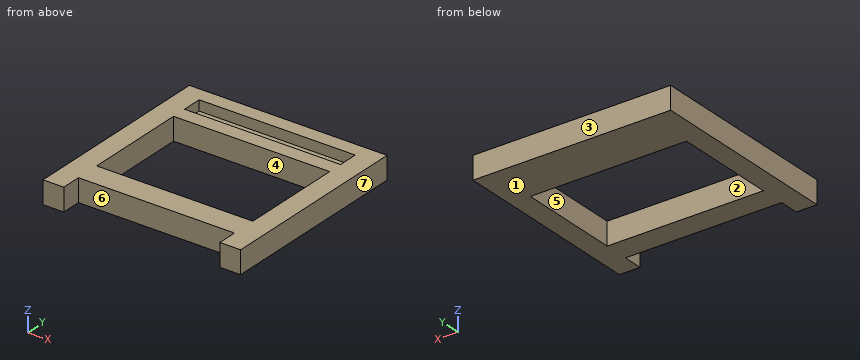
```python
from build123d import *

# Parameters (mm, degrees)
SKETCH1_W           = 15.8
SKETCH1_H           = 10.5
SKETCH1_H_2         = 2
BOSS_EXTRUDE1_DEPTH = 2.3
SKETCH1_2_W         = 15.8
SKETCH1_2_H         = 2
BOSS_EXTRUDE2_DEPTH = 1.25


with BuildPart() as part:
    # Sketch1 → Boss-Extrude1 (new body)
    with BuildSketch(Plane.XY):
        Polygon((0, 0), (0, -2), (2.1, -2), (2.1, 0), (17.9, 0), (17.9, -2), (20, -2), (20, 0), (20, 18), (0, 18), align=None)
        with Locations((10, 7.75)):
            Rectangle(SKETCH1_W, SKETCH1_H, mode=Mode.SUBTRACT)
        with Locations((10, 15.5)):
            Rectangle(SKETCH1_W, SKETCH1_H_2, mode=Mode.SUBTRACT)
    extrude(amount=BOSS_EXTRUDE1_DEPTH)

    # Sketch1<2> → Boss-Extrude2 (add)
    with BuildSketch(Plane.XY):
        with Locations((10, 15.5)):
            Rectangle(SKETCH1_2_W, SKETCH1_2_H)
    extrude(amount=BOSS_EXTRUDE2_DEPTH)


solid = part.part
```
Work out the finished part from the listing and answer in its coordinate system (mm). Face numbers are marked on the shaded views. A direction names the side the tool comes from. Give positions to 0.01 mm unless a question says otherwise; leave off trailing zeros. Write each loop counter-clockwise with the first axis right and the second up, starting at its lowest first coordinate (ties: lowest second). Pieces come first, ordered by that corner, then holes. Notation, with made-up numbers: (-26, -14.5) - (4, -14.5) arc R23 ccw to (4, 16.5) - close; hole circle Ø9 at (-38, -31.75). An arc over 180 degrees is marked (long way). Use one line per item in the form item = value.
1. A cutting plane is placed at A-A (x = 11). Write down the section's boundary in (y, z).
Filled in:
outline = (0, 0) - (2.5, 0) - (2.5, 2.3) - (0, 2.3) - close; (13, 0) - (18, 0) - (18, 2.3) - (16.5, 2.3) - (16.5, 1.25) - (14.5, 1.25) - (14.5, 2.3) - (13, 2.3) - close
2. Determine the mould class of the marked faces 1, 2, 3 and 4 for opening direction Y: released by +Y, released by -Y, zero draft, split by the parting line, or undercut.
Filled in:
face_1 = zero draft
face_2 = undercut
face_3 = released by +Y
face_4 = undercut
3. A cutting plane is placed at D-D (z = 0.6). Write down the section's boundary in (x, y), and give its area (4 significant figures).
Filled in:
outline = (0, -2) - (2.1, -2) - (2.1, 0) - (17.9, 0) - (17.9, -2) - (20, -2) - (20, 18) - (0, 18) - close; hole (2.1, 2.5) - (17.9, 2.5) - (17.9, 13) - (2.1, 13) - close
area = 202.5 mm^2
4. Each of these flat-tipped pins is pushed along its axis until it touches: pin 1 Ø1 at (x, y) = (11, 15.5) entering from +Z; pin 2 Ø1 at (x, y) = (5.5, 14) entering from -Z. Where does it stop, or does it pass through?
Filled in:
pin_1 = 1.25
pin_2 = 0
5. Consider L1, parallel to Y at x = 17.75, z = 2; L2, parallel to Y at x = 7.5, z = 0.7; L3, parallel to X at y = 14.75, z = 2.15. Determine where each line is inside the solid, lowest interval first.
Filled in:
L1 = 0 to 2.5, 13 to 14.5, 16.5 to 18
L2 = 0 to 2.5, 13 to 18
L3 = 0 to 2.1, 17.9 to 20
6. A cutting plane is placed at C-C (z = 2.05). Write down the section's boundary in (x, y).
Filled in:
outline = (0, -2) - (2.1, -2) - (2.1, 0) - (17.9, 0) - (17.9, -2) - (20, -2) - (20, 18) - (0, 18) - close; hole (2.1, 2.5) - (17.9, 2.5) - (17.9, 13) - (2.1, 13) - close; hole (2.1, 14.5) - (17.9, 14.5) - (17.9, 16.5) - (2.1, 16.5) - close
7. For the marked faces 5, 6 and 7, determine the directions among +Z, -Z, +X, -X, +Y, -Y from which every point of the face is accessible in a straight line to the end or side of a thin tool.
Filled in:
face_5 = +Z, -Z
face_6 = +Z, -Z, -Y
face_7 = +Z, -Z, +X, +Y, -Y
8. A cutting plane is placed at B-B (y = 12). Write down the section's boundary in (x, z), and give its area (3 significant figures).
Filled in:
outline = (0, 0) - (2.1, 0) - (2.1, 2.3) - (0, 2.3) - close; (17.9, 0) - (20, 0) - (20, 2.3) - (17.9, 2.3) - close
area = 9.66 mm^2
